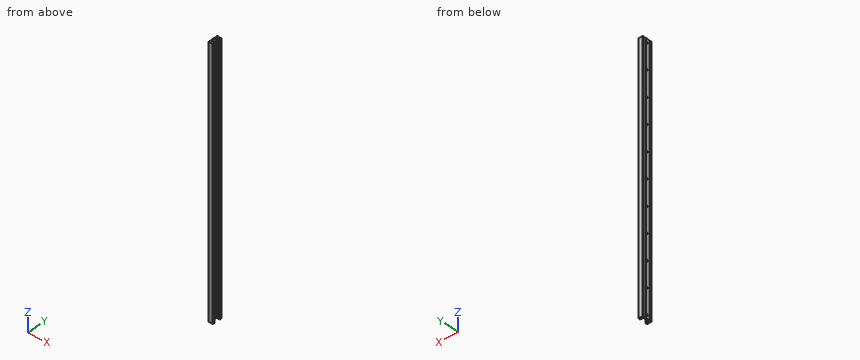
```python
from build123d import *

# Parameters (mm, degrees)
BOSS_EXTRUDE1_DEPTH = 457.2
LPATTERN1_COUNT     = 11
LPATTERN1_PITCH     = 88.9


with BuildPart() as part:
    # Sketch1 → Boss-Extrude1 (new, symmetric)
    with BuildSketch(Plane.XY):
        with BuildLine():
            Line((5.334, 11.303), (5.334, 15.367))
            ThreePointArc((5.334, 15.367), (4.887630735, 16.444630735), (3.81, 16.891))
            Line((3.81, 16.891), (-9.398, 16.891))
            Line((-9.398, 16.891), (-10.414, 15.875))
            Line((-10.414, 15.875), (-10.414, 12.191998878))
            Line((-10.414, 12.191998878), (-9.652, 11.429999439))
            Line((-9.652, 11.429999439), (-9.652, 6.349999439))
            Line((-9.652, 6.349999439), (-10.414, 5.588))
            Line((-10.414, 5.588), (-10.414, -5.588))
            Line((-10.414, -5.588), (-9.652, -6.349999439))
            Line((-9.652, -6.349999439), (-9.652, -11.429999439))
            Line((-9.652, -11.429999439), (-10.414, -12.191998878))
            Line((-10.414, -12.191998878), (-10.414, -15.875))
            Line((-10.414, -15.875), (-9.398, -16.891))
            Line((-9.398, -16.891), (3.81, -16.891))
            ThreePointArc((3.81, -16.891), (4.887630735, -16.444630735), (5.334, -15.367))
            Line((5.334, -15.367), (5.334, -11.303))
            ThreePointArc((5.334, -11.303), (5.185210245, -10.943789755), (4.826, -10.795))
            Line((4.826, -10.795), (2.262739437, -10.795))
            ThreePointArc((2.262739437, -10.795), (0, -9.1694), (-2.262739437, -10.795))
            Line((-2.262739437, -10.795), (-4.318, -10.795))
            ThreePointArc((-4.318, -10.795), (-5.395630735, -10.348630735), (-5.842, -9.271))
            Line((-5.842, -9.271), (-5.842, 9.271))
            ThreePointArc((-5.842, 9.271), (-5.395630735, 10.348630735), (-4.318, 10.795))
            Line((-4.318, 10.795), (-2.262739437, 10.795))
            ThreePointArc((-2.262739437, 10.795), (0, 9.1694), (2.262739437, 10.795))
            Line((2.262739437, 10.795), (4.826, 10.795))
            ThreePointArc((4.826, 10.795), (5.185210245, 10.943789755), (5.334, 11.303))
        make_face()
    extrude(amount=BOSS_EXTRUDE1_DEPTH, both=True)

    # Sketch3 → Cut-Revolve1 (revolve, cut)
    with BuildSketch(Plane.XY.offset(444.5), mode=Mode.PRIVATE) as cut_revolve1_sk:
        Polygon((-5.842, 4.7625), (-8.0518, 4.7625), (-8.0518, 2.4638), (-10.414, 2.4638), (-10.414, 0), (-5.842, 0), align=None)
    cut_revolve1 = revolve(cut_revolve1_sk.sketch.rotate(Axis((-10.414, 0, 444.5), (1, 0, 0)), 180), axis=Axis((-10.414, 0, 444.5), (1, 0, 0)), mode=Mode.SUBTRACT)

    # LPattern1: Cut-Revolve1 ×11
    with Locations(*[(0, 0, -i * LPATTERN1_PITCH) for i in range(1, LPATTERN1_COUNT)]):
        add(cut_revolve1, mode=Mode.SUBTRACT)


solid = part.part
```
For this review, take the finished solid that the model builds, in its own axes (mm). Coordinates: 2 decimals unless noted, no trailing zeros. Write each loop counter-clockwise with the first axis right and the second up, starting at its lowest first coordinate (ties: lowest second). Pieces come first, ordered by that corner, then holes. Notation, with made-up numbers: (42.5, 54.25) - (58.5, 54.25) arc R9 cw to (58.5, 60.25) - close; hole circle Ø11 at (34, 26.5). An arc over 180 degrees is marked (long way). Answer in a Markdown table with one row per item. Add a question column.
Q1. For probe 1 along Y at (x, z) = (-6.6, -266.7); probe 2 along Y at (x, z) = (-3.25, -55) (3 decimals); probe 3 along Y at (x, z) = (-9.75, 444.5), list the stretches that pass through material, from the lowest coordinate up.
Q2. For P1, Ø8.5, axis at y = 0, z = 355.6, coming from the +X side; P2, Ø3, axis at y = -7.5, z = 116, coming from the +X side; P3, Ø15, axis at y = 0, z = 444.5, coming from the -X side, all flat-tipped, find the tip position at first contact; note any pin that passes through.
Q3. We need section A-A, the plane z = 56.5. State the section outline as (x, y) points (3 decimals).
Answer list:
| question | item | result |
|---|---|---|
| 1 | probe 1 | y = -16.89 to -4.76, 4.76 to 16.89 |
| 1 | probe 2 | y = -16.891 to -10.795, 10.795 to 16.891 |
| 1 | probe 3 | y = -16.54 to -11.53, -6.25 to -2.46, 2.46 to 6.25, 11.53 to 16.54 |
| 2 | P1 | stops at x = -8.05 |
| 2 | P2 | stops at x = -5.84 |
| 2 | P3 | stops at x = -10.41 |
| 3 | outline | (-10.414, -15.875) - (-9.398, -16.891) - (3.81, -16.891) arc R1.524 ccw to (5.334, -15.367) - (5.334, -11.303) arc R0.508 ccw to (4.826, -10.795) - (2.263, -10.795) arc R2.388 ccw to (-2.263, -10.795) - (-4.318, -10.795) arc R1.524 cw to (-5.842, -9.271) - (-5.842, 9.271) arc R1.524 cw to (-4.318, 10.795) - (-2.263, 10.795) arc R2.388 ccw to (2.263, 10.795) - (4.826, 10.795) arc R0.508 ccw to (5.334, 11.303) - (5.334, 15.367) arc R1.524 ccw to (3.81, 16.891) - (-9.398, 16.891) - (-10.414, 15.875) - (-10.414, 12.192) - (-9.652, 11.43) - (-9.652, 6.35) - (-10.414, 5.588) - (-10.414, -5.588) - (-9.652, -6.35) - (-9.652, -11.43) - (-10.414, -12.192) - close |
